Could you check a few things on this drawing? It's one solid part, dimensions in mm from its lowest x, y, z. A direction names the side the tool comes from. Give positions to 0.01 mm unless a question says otherwise; leave off trailing zeros. Write each loop counter-clockwise with the first axis right and the second up, starting at its lowest first coordinate (ties: lowest second). Pieces come first, ordered by that corner, then holes.
1. Suppose I cut it at C-C (x = 395). Please give me the cut outline in (y, z), and give its area (3 significant figures).
2. Suppose I cut it at B-B (y = 200). Please give me the cut outline in (x, z).
3. Suppose I cut it at A-A (z = 250). Please give me the cut outline in (x, y).
4. I'm going to push flat-ended pins straight in: pin 1 (8 mm diameter, centred on x = 277.5, z = 222, fed in from -Y); pin 2 (4 mm diameter, centred on x = 350, z = 420.5, fed in from +Y); pin 3 (3 mm diameter, centred on x = 208.5, y = 108.5, fed in from +Z). Where does each tip first touch, or does it pass through?
5. Suppose I cut it at D-D (y = 134). Please give me the cut outline in (x, z).
6. Thinking about a two-plate mould opening in Y: for the marked faces 1, 2 and 3, which applies, pulls with the +Y half, pulls with the -Y half, needs draft (parallel to the pull), parting line crosses it, or undercut?
7. If I drill on probe 1 along Y at (x, z) = (327, 450); probe 2 along X at (y, z) = (281, 174.5); probe 3 along X at (y, z) = (210.5, 221.5), over which ranges is the centre line in solid material (lowest first)?
8. On a 3-axis mill with a long thin cutter (end or side, diameter ignored), from which of +Z, -Z, +X, -X, +Y, -Y can I reach the whole of each face in a straight line? I mean the marked faces 4, 5 and 6. Say none if no direction works.
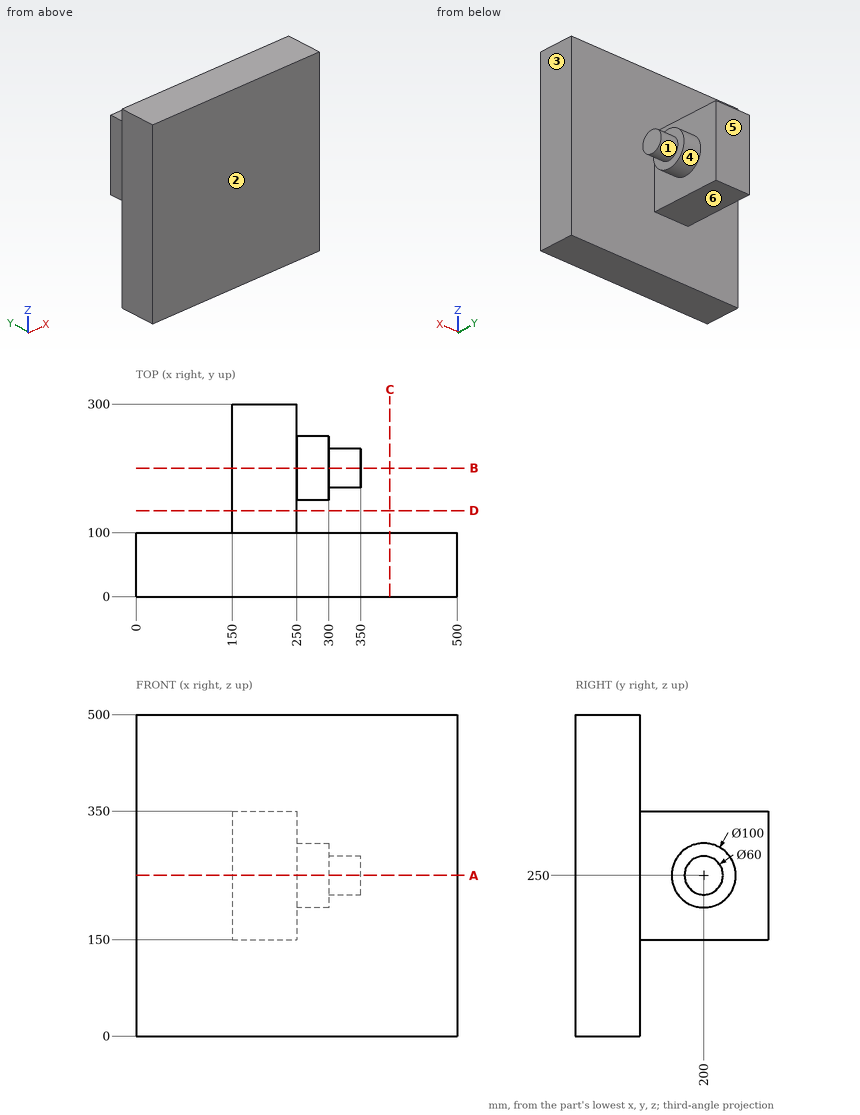
Checks:
1. outline: (0, 0) - (100, 0) - (100, 500) - (0, 500) - close
1. area: 50,000 mm2
2. outline: (150, 150) - (250, 150) - (250, 200) - (300, 200) - (300, 220) - (350, 220) - (350, 280) - (300, 280) - (300, 300) - (250, 300) - (250, 350) - (150, 350) - close
3. outline: (0, 0) - (500, 0) - (500, 100) - (250, 100) - (250, 150) - (300, 150) - (300, 170) - (350, 170) - (350, 230) - (300, 230) - (300, 250) - (250, 250) - (250, 300) - (150, 300) - (150, 100) - (0, 100) - close
4. pin 1: stops at y = 0
4. pin 2: stops at y = 100
4. pin 3: stops at z = 350
5. outline: (150, 150) - (250, 150) - (250, 350) - (150, 350) - close
6. face 1: undercut
6. face 2: pulls with the -Y half
6. face 3: needs draft
7. probe 1: y = 0 to 100
7. probe 2: x = 150 to 250
7. probe 3: x = 150 to 300
8. face 4: +X
8. face 5: +Z, -Z, +X, -X, +Y
8. face 6: -Z, +X, -X, +Y
